Here's how the part is built. I have some questions about the finished solid (model axes, mm). A direction names the side the tool comes from. Give positions to 0.01 mm unless a question says otherwise; leave off trailing zeros. Return JSON: item names as keys, results as strings. Group by question number.
(1) If we mould it in two halves opening along X, with no side actions, what happens to faces 5 (the flat face through (22, 22.225, 0)), 6 (the cylindrical face through (2.22, 13.43, 33.58)), 7 (the flat face through (-16, 19.05, -2))? For each: released by +X, released by -X, zero draft, split by the parting line, or undercut.
(2) For P1, Ø2, axis at x = -15, z = -1, coming from the -Y side; P2, Ø4, axis at x = -12, y = 2.5, coming from the -Z side (3 decimals); P3, Ø3.5, axis at y = 20, z = 7, coming from the +X side; P4, Ø7, axis at y = 15, z = -3.5, coming from the -X side (3 decimals), each with a flat end and sliding along its axis, tell me the tip position at first contact or that it passes through.
(3) I need wall thicknesses on probe 1 along Z at (x, y) = (0, 10.25) (3 decimals); probe 2 along X at (y, z) = (11.5, -0.5); probe 3 along Y at (x, z) = (22, 13) (3 decimals). Which ranges of each line are inside material? Lowest first, please. Write a range as [from, to].
(4) On a 3-axis mill with a long thin cutter (end or side, diameter ignored), from which of +Z, -Z, +X, -X, +Y, -Y can I reach the whole of each face in a straight line? I mean faces 1 (the flat face through (0, 21, -25.718)), 2 (the flat face through (15.24, 16, 0)), 3 (the flat face through (18, 0, 25)), 4 (the flat face through (20, 12.7, 0)). Say none if no direction works.
Autodesk Inventor part; units mm, degrees
ref_plane "YZ Plane" through (0, 0, 0) normal (1, 0, 0) x (0, 1, 0)
ref_plane "XZ Plane" through (0, 0, 0) normal (0, 1, 0) x (-1, 0, 0)
ref_plane "XY Plane" through (0, 0, 0) normal (0, 0, 1) x (1, 0, 0)
sketch "Sketch1" plane through (0, 0, 0) normal (0, 1, 0) x (-1, 0, 0)
  circle A0 centre (0, 0) radius 33.655
  circle A1 centre (0, 0) radius 30.48
  dimension "d0" = 67.31
  dimension "d1" = 60.96
extrude "Extrusion1" add sketch "Sketch1" along normal blind 12.7
sketch "Sketch2" plane through (0, 12.7, 0) normal (0, 1, 0) x (1, 0, 0)
  circle A0 centre (0, 0) radius 33.655
extrude "Extrusion2" add sketch "Sketch2" along normal blind 9.525
sketch "Sketch3" plane through (0, 22.225, 0) normal (0, 1, 0) x (1, 0, 0)
  line L0 (18.0975, -25.7175) -> (-18.0975, -25.7175)
  line L1 (-18.0975, -25.7175) -> (-18.0975, 25.7175)
  line L2 (-18.0975, 25.7175) -> (18.0975, 25.7175)
  line L3 (18.0975, 25.7175) -> (18.0975, -25.7175)
  line L4 (18.0975, -25.7175) -> (-18.0975, 25.7175) construction
  line L5 (-18.0975, -25.7175) -> (18.0975, 25.7175) construction
  point P0 (0, 0)
  dimension "d6" = 36.195
  dimension "d7" = 51.435
extrude "Extrusion3" cut sketch "Sketch3" against normal blind 3.175
sketch "Sketch4" plane through (0, 19.05, 0) normal (0, 1, 0) x (1, 0, 0)
  line L0 (15.24, -22.86) -> (-15.24, -22.86)
  line L1 (-15.24, -22.86) -> (-15.24, 22.86)
  line L2 (-15.24, 22.86) -> (15.24, 22.86)
  line L3 (15.24, 22.86) -> (15.24, -22.86)
  line L4 (15.24, -22.86) -> (-15.24, 22.86) construction
  line L5 (-15.24, -22.86) -> (15.24, 22.86) construction
  point P0 (0, 0)
  dimension "d10" = 30.48
  dimension "d11" = 45.72
extrude "Extrusion4" cut sketch "Sketch4" against normal through all
properties part number "Upper Collar"
Values:
{
 "1": {"face 5": "zero draft", "face 6": "split by the parting line", "face 7": "undercut"},
 "2": {"P1": "y = 12.7", "P2": "z = -32.135", "P3": "x = 33.24", "P4": "x = -33.655"},
 "3": {"probe 1": "[-33.655, -30.48], [30.48, 33.655]", "probe 2": "[-33.65, -30.48], [30.48, 33.65]", "probe 3": "[12.7, 22.225]"},
 "4": {"face 1": "+Y", "face 2": "+Y, -Y", "face 3": "+Z, -Z, +X, -X, -Y", "face 4": "-Y"}
}
